Part model, mm, in its own coordinate system. Face numbers are marked on the shaded views. A direction names the side the tool comes from. Give positions to 0.01 mm unless a question says otherwise; leave off trailing zeros. Write each loop counter-clockwise with the first axis right and the second up, starting at its lowest first coordinate (ties: lowest second). Pieces come first, ordered by that corner, then holes. Notation, with made-up numbers: (6, -4.75) - (63, -4.75) arc R13 ccw to (63, 17.25) - close; hole circle Ø7 at (-35.75, 78). An arc over 180 degrees is marked (long way). Answer as a JSON object with one key per item and string values. Group by question number.
```python
from build123d import *

# Parameters (mm, degrees)
SKETCH_1_R               = 22.5
SKETCH_1_R_2             = 10
EXTRUDE_1_DEPTH          = 6
SKETCH1_OUTSIDE_W        = 59.952
SKETCH1_OUTSIDE_H        = 59.952
SKETCH1_OUTSIDE_R        = 18.5
CUT_EXTRUDE1_DEPTH       = 1
M3_TAPPED_HOLE1_D        = 2.5
PATTERN_CIRCULAR_1_COUNT = 6
CHAMFER_1_SIZE           = 0.5


with BuildPart() as part:
    # Sketch 1 → Extrude 1 (new, symmetric)
    with BuildSketch(Plane.XY):
        Circle(SKETCH_1_R)
        Circle(SKETCH_1_R_2, mode=Mode.SUBTRACT)
    extrude(amount=EXTRUDE_1_DEPTH, both=True)

    # Sketch1 outside → Cut-Extrude1 (cut)
    with BuildSketch(Plane(origin=(0, 0, -6), x_dir=(-1, 0, 0), z_dir=(0, 0, -1))):
        Rectangle(SKETCH1_OUTSIDE_W, SKETCH1_OUTSIDE_H)
        Circle(SKETCH1_OUTSIDE_R, mode=Mode.SUBTRACT)
    cut_extrude1 = extrude(amount=-CUT_EXTRUDE1_DEPTH, mode=Mode.SUBTRACT)

    # Mirror1: Cut-Extrude1 across plane
    add(cut_extrude1.mirror(Plane.XY), mode=Mode.SUBTRACT)

    # M3 Tapped Hole1 (through all)
    with Locations(Plane.XY.offset(6)):
        with Locations((0, 14)):
            m3_tapped_hole1 = Hole(M3_TAPPED_HOLE1_D / 2)

    # Pattern Circular 1: M3 Tapped Hole1 ×6 about axis
    pattern_circular_1_axis = Axis((0, 0, 0), (0, 0, 1))
    for i in range(1, PATTERN_CIRCULAR_1_COUNT):
        add(m3_tapped_hole1.rotate(pattern_circular_1_axis, i * 360 / PATTERN_CIRCULAR_1_COUNT), mode=Mode.SUBTRACT)

    # Chamfer 1
    chamfer_1_edges = [part.edges().sort_by_distance(p)[0] for p in [
        (18.5, 0, -6),
        (18.5, 0, 6),
        (-10, 0, -6),
        (-10, 0, 6),
    ]]
    chamfer(chamfer_1_edges, length=CHAMFER_1_SIZE)


solid = part.part
```
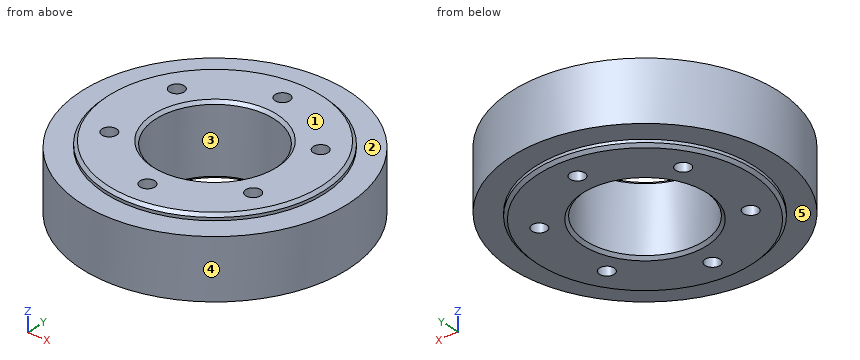
1) Saw through at C-C (z = -1). List the corners of the cut face in (x, y), and give its area (3 significant figures).
2) Which spindle directions (+Z, -Z, +X, -X, +Y, -Y) get a long thin tool onto all of the face, cutting with end or side? Do the marked faces 1 and 2. Say none if no direction does.
3) Saw through at A-A (x = 0). State how many separate pieces and enclosed holes the cut face has, and give its area (3 significant figures).
4) Saw through at B-B (y = 0). List the corners of the cut face in (x, z).
5) Drill centre lines: line 1 along Y through (x, z) = (-12.5, 0.5); line 2 along Y through (x, z) = (13, 4.5); line 3 along Z through (x, y) = (15, 13). Where is each one in solid material? Low to high. Write a range as from..to.
6) Drop flat-ended pins along their axis: P1, Ø1.5, axis at y = 8, z = -2, coming from the +X side; P2, Ø5, axis at y = -7.5, z = -1, coming from the -X side; P3, Ø4, axis at x = 11.5, z = 4.5, coming from the +Y side. Give the stop position or say it passes through.
7) Two-plate mould, pull along Y, no slides. Class the marked faces 3, 4 and 5: +Y half, -Y half, draft (parallel to the pull), parting line (faces both ways), or undercut.
Checks:
{
 "1": {"outline": "circle Ø45 at (0, 0); hole circle Ø2.5 at (-12.12, -7); hole circle Ø2.5 at (-12.12, 7); hole circle Ø20 at (0, 0); hole circle Ø2.5 at (0, -14); hole circle Ø2.5 at (0, 14); hole circle Ø2.5 at (12.12, -7); hole circle Ø2.5 at (12.12, 7)", "area": "1,250 mm2"},
 "2": {"face 1": "+Z, +X, -X, +Y, -Y", "face 2": "+Z"},
 "3": {"separate pieces": "4", "enclosed holes": "0", "area": "223 mm2"},
 "4": {"outline": "(-22.5, -5) - (-18.5, -5) - (-18.5, -5.5) - (-18, -6) - (-10.5, -6) - (-10, -5.5) - (-10, 5.5) - (-10.5, 6) - (-18, 6) - (-18.5, 5.5) - (-18.5, 5) - (-22.5, 5) - close; (10, -5.5) - (10.5, -6) - (18, -6) - (18.5, -5.5) - (18.5, -5) - (22.5, -5) - (22.5, 5) - (18.5, 5) - (18.5, 5.5) - (18, 6) - (10.5, 6) - (10, 5.5) - close"},
 "5": {"line 1": "-18.71..-8.19, -5.81..5.81, 8.19..18.71", "line 2": "-18.36..-7.89, -6.11..6.11, 7.89..18.36", "line 3": "-5..5"},
 "6": {"P1": "x = 21.3", "P2": "x = -21.94", "P3": "y = 20.4"},
 "7": {"face 3": "undercut", "face 4": "parting line", "face 5": "draft"}
}
